```python
from build123d import *

# Parameters (mm, degrees)
SKETCH1_R           = 10.65
BOSS_EXTRUDE1_DEPTH = 4
CUT_EXTRUDE2_START  = -2
SKETCH4_R           = 11.65
SKETCH4_R_2         = 10.65
CUT_EXTRUDE2_DEPTH  = 2
CUT_EXTRUDE3_START  = -0.25
SKETCH5_R           = 11.65
SKETCH5_R_2         = 11.15
CUT_EXTRUDE3_DEPTH  = 0.25
FILLET1_R           = 0.1
BOSS_EXTRUDE3_DEPTH = 30
CUT_EXTRUDE6_START  = -30
SKETCH12_R          = 10.65
CUT_EXTRUDE6_DEPTH  = 30
CUT_EXTRUDE7_DEPTH  = 30
SKETCH14_R          = 1
CUT_EXTRUDE8_DEPTH  = 30
SKETCH15_R          = 1
CUT_EXTRUDE9_DEPTH  = 30


with BuildPart() as part:
    # Sketch1 → Boss-Extrude1 (new body)
    with BuildSketch(Plane(origin=(0, 0, 0), x_dir=(0, 0, -1), z_dir=(1, 0, 0))):
        Polygon((44.818066557, 64.750067007), (49.818066557, 64.750067007), (49.818066557, 34.750067007), (44.818066557, 34.750067007), (-35.181933443, 34.750067007), (-40.181933443, 34.750067007), (-40.181933443, 64.750067007), (-35.181933443, 64.750067007), align=None)
        with Locations((4.818066557, 49.750067007)):
            Circle(SKETCH1_R, mode=Mode.SUBTRACT)
    extrude(amount=BOSS_EXTRUDE1_DEPTH)

    # Sketch4 → Cut-Extrude2 (cut)
    with BuildSketch(Plane(origin=(4, 0, 0), x_dir=(0, 0, -1), z_dir=(1, 0, 0)).offset(CUT_EXTRUDE2_START)):
        with Locations((4.818066557, 49.750067007)):
            Circle(SKETCH4_R)
        with Locations((4.818066557, 49.750067007)):
            Circle(SKETCH4_R_2, mode=Mode.SUBTRACT)
    extrude(amount=CUT_EXTRUDE2_DEPTH, mode=Mode.SUBTRACT)

    # Sketch5 → Cut-Extrude3 (cut)
    with BuildSketch(Plane(origin=(2, 0, 0), x_dir=(0, 0, -1), z_dir=(1, 0, 0)).offset(CUT_EXTRUDE3_START)):
        with Locations((4.818066557, 49.750067007)):
            Circle(SKETCH5_R)
        with Locations((4.818066557, 49.750067007)):
            Circle(SKETCH5_R_2, mode=Mode.SUBTRACT)
    extrude(amount=CUT_EXTRUDE3_DEPTH, mode=Mode.SUBTRACT)

    # Fillet1
    fillet1_edges = [part.edges().sort_by_distance(p)[0] for p in [
        (1.75, 49.750067007, 6.331933443),
    ]]
    fillet(fillet1_edges, radius=FILLET1_R)

    # Sketch11 → Boss-Extrude3 (add)
    with BuildSketch(Plane(origin=(0, 64.750067007, 0), x_dir=(1, 0, 0), z_dir=(0, 1, 0))):
        with BuildLine():
            Line((0, 49.818066557), (0, -40.181933443))
            Line((0, -40.181933443), (-18.584993082, -40.181933443))
            ThreePointArc((-18.584993082, -40.181933443), (-1, 4.818066557), (-18.584993082, 49.818066557))
            Line((-18.584993082, 49.818066557), (0, 49.818066557))
        make_face()
    extrude(amount=-BOSS_EXTRUDE3_DEPTH)

    # Sketch12 → Cut-Extrude6 (cut)
    with BuildSketch(Plane(origin=(0, 0, 0), x_dir=(0, 0, -1), z_dir=(1, 0, 0)).offset(CUT_EXTRUDE6_START)):
        with Locations((4.818066557, 49.750067007)):
            Circle(SKETCH12_R)
    extrude(amount=CUT_EXTRUDE6_DEPTH, mode=Mode.SUBTRACT)

    # Sketch13 → Cut-Extrude7 (cut)
    with BuildSketch(Plane(origin=(0, 64.750067007, 0), x_dir=(1, 0, 0), z_dir=(0, 1, 0))):
        Polygon((-12.938744811, 49.818066557), (4, 32.879321746), (4, 49.818066557), align=None)
        Polygon((-12.938744811, -40.181933443), (4, -23.243188631), (4, -40.181933443), align=None)
    extrude(amount=-CUT_EXTRUDE7_DEPTH, mode=Mode.SUBTRACT)

    # Sketch14 → Cut-Extrude8 (cut)
    with BuildSketch(Plane(origin=(-109.620613418, 0, 136.863802049), x_dir=(-0.7071067811865562, 0, 0.7071067811865388), z_dir=(-0.7071067811865388, 0, -0.7071067811865562))):
        with Locations(Location((-148.70631114, 57.250067007, 0), (0, 0, 180))):
            Circle(SKETCH14_R)
        with Locations(Location((-148.70631114, 42.250067007, 0), (0, 0, 180))):
            Circle(SKETCH14_R)
    extrude(amount=CUT_EXTRUDE8_DEPTH, mode=Mode.SUBTRACT)

    # Sketch15 → Cut-Extrude9 (cut)
    with BuildSketch(Plane(origin=(18.539804897, 0, -18.339516848), x_dir=(0.7071067811865562, 0, 0.7071067811865388), z_dir=(-0.7071067811865388, 0, 0.7071067811865562))):
        with Locations(Location((-32.398265563, 57.250067007, 0), (0, 0, 180))):
            Circle(SKETCH15_R)
        with Locations(Location((-32.398265563, 42.250067007, 0), (0, 0, 180))):
            Circle(SKETCH15_R)
    extrude(amount=CUT_EXTRUDE9_DEPTH, mode=Mode.SUBTRACT)


solid = part.part
```
Here's how the part is built. I have some questions about the finished solid (model axes, mm). A direction names the side the tool comes from. Coordinates: 2 decimals unless noted, no trailing zeros. Write each loop counter-clockwise with the first axis right and the second up, starting at its lowest first coordinate (ties: lowest second). Pieces come first, ordered by that corner, then holes. Notation, with made-up numbers: (-35, 31.25) - (18, 31.25) arc R7 cw to (18, 42.25) - close; hole circle Ø5 at (65, -24.75). An arc over 180 degrees is marked (long way). One line per item, written item: value.
1) I'm going to push flat-ended pins straight in: P1, Ø8, axis at y = 57, z = -14.5, coming from the -X side; P2, Ø5, axis at y = 56.5, z = 5.5, coming from the -X side; P3, Ø2, axis at x = -2, y = 54.5, coming from the +Z side. Where does each tip first touch, or does it pass through?
Model answer:
P1: stops at x = -2.43
P2: stops at x = -2.25
P3: stops at z = 30.24
2) On a 3-axis mill with a long thin cutter (end or side, diameter ignored), from which of +Z, -Z, +X, -X, +Y, -Y can I reach the whole of each face in a straight line? I mean faces 1 (the cylindrical face through (2.859, 39.415, -10.194)), 2 (the cylindrical face through (-6.226, 57.633, 28.649)). Say none if no direction works.
Model answer:
face 1: +X
face 2: none
3) Suppose I cut it at D-D on z = 18.5. Write out the boundary of the cut face in (x, y), and give its area (3 significant figures).
Model answer:
outline: (-5.23, 34.75) - (4, 34.75) - (4, 64.75) - (-5.23, 64.75) - close
area: 277 mm²
4) We'd pull the mould along Y, two halves only. Please class faces 3 (the flat face through (-4.588, 49.96, 31.831)), 4 (the cylindrical face through (-6.226, 42.633, 28.649)), 5 (the flat face through (0, 34.75, -5)), 6 (the cylindrical face through (-6.088, 57.206, -38.117)): pulls with the +Y half, pulls with the -Y half, needs draft (parallel to the pull), parting line crosses it, or undercut.
Model answer:
face 3: needs draft
face 4: undercut
face 5: pulls with the -Y half
face 6: undercut
5) I need wall thicknesses on line 1 along Z through (x, y) = (-9.75, 50.5); line 2 along Z through (x, y) = (-1.25, 55); line 3 along X through (y, z) = (51, -24). Which ranges of each line are inside material? Lowest first, please.
Model answer:
line 1: z = -46.63 to -37.76, 28.12 to 36.99
line 2: z = -38.13 to -14.08, 4.45 to 28.49
line 3: x = -3.83 to 4
6) Suppose I cut it at B-B on x = -7.5. State how many separate pieces and enclosed holes the cut face has, and give its area (3 significant figures).
Model answer:
separate pieces: 2
enclosed holes: 4
area: 637 mm²
7) Suppose I cut it at C-C on x = 0.5. Write out the boundary of the cut face in (y, z), and give its area (3 significant figures).
Model answer:
outline: (34.75, -36.38) - (64.75, -36.38) - (64.75, 26.74) - (34.75, 26.74) - close; hole circle Ø21.3 at (49.75, -4.82)
area: 1,540 mm²
8) Suppose I cut it at A-A on x = -17. Write out the boundary of the cut face in (y, z), and give its area (3 significant figures).
Model answer:
outline: (34.75, -49.82) - (64.75, -49.82) - (64.75, -48.04) - (34.75, -48.04) - close; (34.75, 38.4) - (64.75, 38.4) - (64.75, 40.18) - (34.75, 40.18) - close
area: 107 mm²
